Source: CAD feature listing. Evaluate the final solid. Frame: model axes, mm. Coordinates: 2 decimals unless noted, no trailing zeros. Order: outer loops, then holes, each group sorted by start corner. A loop starts at its lowest first (then second) coordinate and runs counter-clockwise, first axis right, second up.
```python
from build123d import *

# Parameters (mm, degrees)
SKETCH1_W           = 250
SKETCH1_H           = 250
BOSS_EXTRUDE1_DEPTH = 2.5
CUT_EXTRUDE1_REACH  = 7
SKETCH2_W           = 100
SKETCH2_H           = 10
CUT_EXTRUDE2_REACH  = 7
SKETCH4_R           = 1.5
FILLET1_R           = 30


with BuildPart() as part:
    # Sketch1 → Boss-Extrude1 (new body, symmetric)
    with BuildSketch(Plane(origin=(0, 0, 0), x_dir=(1, 0, 0), z_dir=(0, 1, 0))):
        Rectangle(SKETCH1_W, SKETCH1_H)
    extrude(amount=BOSS_EXTRUDE1_DEPTH, both=True)

    # Sketch2 → Cut-Extrude1 (cut, up to next)
    with BuildSketch(Plane(origin=(0, 2.5, 0), x_dir=(1, 0, 0), z_dir=(0, 1, 0)), mode=Mode.PRIVATE) as cut_extrude1_sk1:
        with Locations((0, 95.139170266)):
            Rectangle(SKETCH2_W, SKETCH2_H)
    cut_extrude1_tool1 = extrude(cut_extrude1_sk1.sketch, amount=-CUT_EXTRUDE1_REACH, mode=Mode.PRIVATE) & part.part
    add(cut_extrude1_tool1.solids().sort_by_distance((0, 2.5, -95.13917))[0], mode=Mode.SUBTRACT)

    # Sketch4 → Cut-Extrude2 (cut, up to next)
    with BuildSketch(Plane(origin=(0, 2.5, 0), x_dir=(1, 0, 0), z_dir=(0, 1, 0)), mode=Mode.PRIVATE) as cut_extrude2_sk1:
        with Locations((-108, 108)):
            Circle(SKETCH4_R)
    cut_extrude2_tool1 = extrude(cut_extrude2_sk1.sketch, amount=-CUT_EXTRUDE2_REACH, mode=Mode.PRIVATE) & part.part
    add(cut_extrude2_tool1.solids().sort_by_distance((-108, 2.5, -108))[0], mode=Mode.SUBTRACT)
    # Sketch4 → Cut-Extrude2 (cut, up to next)
    with BuildSketch(Plane(origin=(0, 2.5, 0), x_dir=(1, 0, 0), z_dir=(0, 1, 0)), mode=Mode.PRIVATE) as cut_extrude2_sk2:
        with Locations((0, 108)):
            Circle(SKETCH4_R)
    cut_extrude2_tool2 = extrude(cut_extrude2_sk2.sketch, amount=-CUT_EXTRUDE2_REACH, mode=Mode.PRIVATE) & part.part
    add(cut_extrude2_tool2.solids().sort_by_distance((0, 2.5, -108))[0], mode=Mode.SUBTRACT)
    # Sketch4 → Cut-Extrude2 (cut, up to next)
    with BuildSketch(Plane(origin=(0, 2.5, 0), x_dir=(1, 0, 0), z_dir=(0, 1, 0)), mode=Mode.PRIVATE) as cut_extrude2_sk3:
        with Locations((108, 108)):
            Circle(SKETCH4_R)
    cut_extrude2_tool3 = extrude(cut_extrude2_sk3.sketch, amount=-CUT_EXTRUDE2_REACH, mode=Mode.PRIVATE) & part.part
    add(cut_extrude2_tool3.solids().sort_by_distance((108, 2.5, -108))[0], mode=Mode.SUBTRACT)
    # Sketch4 → Cut-Extrude2 (cut, up to next)
    with BuildSketch(Plane(origin=(0, 2.5, 0), x_dir=(1, 0, 0), z_dir=(0, 1, 0)), mode=Mode.PRIVATE) as cut_extrude2_sk4:
        with Locations((108, -108)):
            Circle(SKETCH4_R)
    cut_extrude2_tool4 = extrude(cut_extrude2_sk4.sketch, amount=-CUT_EXTRUDE2_REACH, mode=Mode.PRIVATE) & part.part
    add(cut_extrude2_tool4.solids().sort_by_distance((108, 2.5, 108))[0], mode=Mode.SUBTRACT)
    # Sketch4 → Cut-Extrude2 (cut, up to next)
    with BuildSketch(Plane(origin=(0, 2.5, 0), x_dir=(1, 0, 0), z_dir=(0, 1, 0)), mode=Mode.PRIVATE) as cut_extrude2_sk5:
        with Locations((0, -108)):
            Circle(SKETCH4_R)
    cut_extrude2_tool5 = extrude(cut_extrude2_sk5.sketch, amount=-CUT_EXTRUDE2_REACH, mode=Mode.PRIVATE) & part.part
    add(cut_extrude2_tool5.solids().sort_by_distance((0, 2.5, 108))[0], mode=Mode.SUBTRACT)
    # Sketch4 → Cut-Extrude2 (cut, up to next)
    with BuildSketch(Plane(origin=(0, 2.5, 0), x_dir=(1, 0, 0), z_dir=(0, 1, 0)), mode=Mode.PRIVATE) as cut_extrude2_sk6:
        with Locations((-108, -108)):
            Circle(SKETCH4_R)
    cut_extrude2_tool6 = extrude(cut_extrude2_sk6.sketch, amount=-CUT_EXTRUDE2_REACH, mode=Mode.PRIVATE) & part.part
    add(cut_extrude2_tool6.solids().sort_by_distance((-108, 2.5, 108))[0], mode=Mode.SUBTRACT)

    # Fillet1
    fillet1_edges = [part.edges().sort_by_distance(p)[0] for p in [
        (125, 0, 125),
        (-125, 0, 125),
        (-125, 0, -125),
        (125, 0, -125),
    ]]
    fillet(fillet1_edges, radius=FILLET1_R)


solid = part.part
```
1. Section query A-A, the plane x = -42.5. Output: boundary loops of the cut face in (y, z).
2. Material intervals for line 1 along Z through (x, y) = (0, 0.1); line 2 along X through (y, z) = (-0.35, -108); line 3 along Z through (x, y) = (108, 0.25), sorted ascending.
3. Section query B-B, the plane y = 1.4. Output: boundary loops of the cut face in (x, z).
4. Draft query along Y for faces 1 (the cylindrical face through (115.979, -0.035, -116.445)), 2 (the flat face through (-2, 2.5, -2)), 3 (the flat face through (-2, -2.5, -2)). Return one class per face: +Y half, -Y half, draft (parallel to the pull), parting line (faces both ways), or undercut.
5. Contact query for flat-ended pins moving along their axis: P1, Ø4, axis at x = 0, z = -108, coming from the -Y side; P2, Ø1.5, axis at y = 1, z = -96, coming from the +X side; P3, Ø1.8, axis at x = -108, z = -108, coming from the -Y side. Output: stop coordinate, or through.
Answer key:
1. outline: (-2.5, -125) - (2.5, -125) - (2.5, -100.14) - (-2.5, -100.14) - close; (-2.5, -90.14) - (2.5, -90.14) - (2.5, 125) - (-2.5, 125) - close
2. line 1: z = -125 to -109.5, -106.5 to -100.14, -90.14 to 106.5, 109.5 to 125
2. line 2: x = -122.04 to -109.5, -106.5 to -1.5, 1.5 to 106.5, 109.5 to 122.04
2. line 3: z = -122.04 to -109.5, -106.5 to 106.5, 109.5 to 122.04
3. outline: (-125, -95) arc R30 ccw to (-95, -125) - (95, -125) arc R30 ccw to (125, -95) - (125, 95) arc R30 ccw to (95, 125) - (-95, 125) arc R30 ccw to (-125, 95) - close; hole circle Ø3 at (-108, -108); hole circle Ø3 at (-108, 108); hole (-50, -100.14) - (50, -100.14) - (50, -90.14) - (-50, -90.14) - close; hole circle Ø3 at (0, -108); hole circle Ø3 at (0, 108); hole circle Ø3 at (108, -108); hole circle Ø3 at (108, 108)
4. face 1: draft
4. face 2: +Y half
4. face 3: -Y half
5. P1: stops at y = -2.5
5. P2: stops at x = 125
5. P3: passes through
